Model file for the job. Use its own axes, mm. A direction names the side the tool comes from. Give positions to 0.01 mm unless a question says otherwise; leave off trailing zeros. Write each loop counter-clockwise with the first axis right and the second up, starting at its lowest first coordinate (ties: lowest second). Pieces come first, ordered by that corner, then holes.
```python
from build123d import *

# Parameters (mm, degrees)
SKETCH1_R             = 10.5
SKETCH1_R_2           = 3
EXTRUDE1_DEPTH        = 46.5
SKETCH1_3_R           = 3
CUT_EXTRUDE1_DEPTH    = 49.813420286
CUT_EXTRUDE4_DEPTH    = 8.5
CUT_EXTRUDE6_START    = -37
SKETCH6_R             = 10.5
SKETCH6_R_2           = 6
CUT_EXTRUDE6_DEPTH    = 37
CUT_EXTRUDE7_START    = -1
SKETCH7_R             = 10.5
SKETCH7_R_2           = 7.5
CUT_EXTRUDE7_DEPTH    = 1
M4X0_7_TAPPED_HOLE1_D = 3
SKETCH8_OUTSIDE_W     = 33.82
SKETCH8_OUTSIDE_H     = 30.82
CUT_EXTRUDE8_DEPTH    = 30
FILLET1_R             = 0.5
CHAMFER1_SIZE         = 0.5
FILLET2_R             = 0.3
CHAMFER2_SIZE         = 1


with BuildPart() as part:
    # Sketch1 → Extrude1 (new body)
    # profile 1 of 2: a face of its own
    with BuildSketch(Plane.XY):
        Circle(SKETCH1_R)
        Circle(SKETCH1_R_2, mode=Mode.SUBTRACT)
    # profile 2 of 2: a face of its own
    with BuildSketch(Plane.XY):
        Circle(SKETCH1_R_2)
    extrude(amount=-EXTRUDE1_DEPTH)

    # Sketch1<3> → Cut-Extrude1 (cut, through all)
    with BuildSketch(Plane.XY):
        Circle(SKETCH1_3_R)
    extrude(amount=-CUT_EXTRUDE1_DEPTH, mode=Mode.SUBTRACT)

    # Sketch4 → Cut-Extrude4 (cut)
    with BuildSketch(Plane.XY):
        with BuildLine():
            Line((-10.24499878, 2.3), (10.24499878, 2.3))
            ThreePointArc((10.24499878, 2.3), (0, 10.5), (-10.24499878, 2.3))
        make_face()
    extrude(amount=-CUT_EXTRUDE4_DEPTH, mode=Mode.SUBTRACT)

    # Sketch6 → Cut-Extrude6 (cut)
    with BuildSketch(Plane(origin=(0, 0, -46.5), x_dir=(1, 0, 0), z_dir=(0, 0, -1)).offset(CUT_EXTRUDE6_START)):
        Circle(SKETCH6_R)
        with Locations(Location((0, 0, 0), (0, 0, 270))):
            Circle(SKETCH6_R_2, mode=Mode.SUBTRACT)
    extrude(amount=CUT_EXTRUDE6_DEPTH, mode=Mode.SUBTRACT)

    # Sketch7 → Cut-Extrude7 (cut)
    with BuildSketch(Plane(origin=(0, 0, -9.5), x_dir=(1, 0, 0), z_dir=(0, 0, -1)).offset(CUT_EXTRUDE7_START)):
        Circle(SKETCH7_R)
        with Locations(Location((0, 0, 0), (0, 0, 270))):
            Circle(SKETCH7_R_2, mode=Mode.SUBTRACT)
    extrude(amount=CUT_EXTRUDE7_DEPTH, mode=Mode.SUBTRACT)

    # M4x0.7 Tapped Hole1 (through all)
    with Locations(Plane(origin=(6.25, 2.3, -4.25), x_dir=(0, 0, 1), z_dir=(0, 1, 0))):
        with Locations((0, 0), (0, -12.5)):
            Hole(M4X0_7_TAPPED_HOLE1_D / 2)

    # Sketch8 outside → Cut-Extrude8 (cut)
    with BuildSketch(Plane(origin=(0, 0, -46.5), x_dir=(1, 0, 0), z_dir=(0, 0, -1))):
        with Locations((0, 1.5)):
            Rectangle(SKETCH8_OUTSIDE_W, SKETCH8_OUTSIDE_H)
        Polygon((0, 5.773502692), (-5, 2.886751346), (-5, -2.886751346), (0, -5.773502692), (5, -2.886751346), (5, 2.886751346), align=None, mode=Mode.SUBTRACT)
    extrude(amount=-CUT_EXTRUDE8_DEPTH, mode=Mode.SUBTRACT)

    # Fillet1
    fillet1_edges = [part.edges().sort_by_distance(p)[0] for p in [
        (5, -2.886751346, -31.5),
        (5, 2.886751346, -31.5),
        (0, 5.773502692, -31.5),
        (-5, 2.886751346, -31.5),
        (-5, -2.886751346, -31.5),
        (0, -5.773502692, -31.5),
    ]]
    fillet(fillet1_edges, radius=FILLET1_R)

    # Chamfer1
    chamfer1_edges = [part.edges().sort_by_distance(p)[0] for p in [
        (-2.5, -4.330127019, -46.5),
        (2.5, -4.330127019, -46.5),
        (-5, 0, -46.5),
        (-2.5, 4.330127019, -46.5),
        (2.5, 4.330127019, -46.5),
        (5, 0, -46.5),
        (0, -5.696152423, -46.5),
        (4.933012702, -2.848076211, -46.5),
        (4.933012702, 2.848076211, -46.5),
        (0, 5.696152423, -46.5),
        (-4.933012702, 2.848076211, -46.5),
        (-4.933012702, -2.848076211, -46.5),
    ]]
    chamfer(chamfer1_edges, length=CHAMFER1_SIZE - 0.0001)  # a hair under: the kernel refuses the full size

    # Sketch12 → Groove for ANSI B27.7 - 3AM1-12, Basic External Retaining Ring1 (revolve, cut)
    with BuildSketch(Plane(origin=(0, 0, 19.370057685), x_dir=(0, 1, 0), z_dir=(-1, 0, 0))):
        with BuildLine():
            Line((5.775, 33.970057685), (7.275, 33.970057685))
            Line((7.275, 33.970057685), (7.275, 35.070057685))
            Line((7.275, 35.070057685), (5.775, 35.070057685))
            ThreePointArc((5.775, 35.070057685), (5.704289322, 35.040768363), (5.675, 34.970057685))
            Line((5.675, 34.970057685), (5.675, 34.070057685))
            ThreePointArc((5.675, 34.070057685), (5.704289322, 33.999347007), (5.775, 33.970057685))
        make_face()
    revolve(axis=Axis((0, 0, 69.359173663), (0, 0, -1)), mode=Mode.SUBTRACT)

    # Fillet2
    fillet2_edges = [part.edges().sort_by_distance(p)[0] for p in [
        (0, -6, -9.5),
        (0, -7.5, -8.5),
    ]]
    fillet(fillet2_edges, radius=FILLET2_R)

    # Chamfer2
    chamfer2_edges = [part.edges().sort_by_distance(p)[0] for p in [
        (0, -10.5, 0),
        (0, -10.5, -8.5),
    ]]
    chamfer(chamfer2_edges, length=CHAMFER2_SIZE)


solid = part.part
```
1. Slice it at A-A, the plane z = -20.5. Write the cut outline in (x, y), and give its area (3 significant figures).
Calculated:
outline: (-5, -2.6) arc R0.5 ccw to (-4.75, -3.03) - (-0.25, -5.63) arc R0.5 ccw to (0.25, -5.63) - (4.75, -3.03) arc R0.5 ccw to (5, -2.6) - (5, 2.6) arc R0.5 ccw to (4.75, 3.03) - (0.25, 5.63) arc R0.5 ccw to (-0.25, 5.63) - (-4.75, 3.03) arc R0.5 ccw to (-5, 2.6) - close; hole circle Ø6 at (0, 0)
area: 58.2 mm2
2. Pin check, flat tips, straight feed: P1, Ø6, axis at y = 0.5, z = -24.5, coming from the +X side; P2, Ø1.6, axis at x = 0.5, y = 4.5, coming from the +Z side; P3, Ø10, axis at x = 5, z = -32.5, coming from the +Y side. Stop position of each tip, or through.
Calculated:
P1: stops at x = 5
P2: stops at z = -8.5
P3: stops at y = 5.7
3. Which spindle directions (+Z, -Z, +X, -X, +Y, -Y) get a long thin tool onto all of the face, cutting with end or side? Do faces 1 (the cylindrical face through (-2.174, 5.242, -15.144)), 2 (the cylindrical face through (1.802, 5.723, -16.094)), 3 (the flat face through (-5, 0, -31)), 4 (the flat face through (0, 4, -8.5)), 5 (the flat face through (-2.469, -4.348, -31.457)). Say none if no direction does.
Calculated:
face 1: none
face 2: -Z
face 3: -Z, -X, +Y, -Y
face 4: +Z, +X, -X, +Y
face 5: -Z, -X, -Y
4. Slice it at B-B, the plane y = 0. State how many separate pieces and enclosed holes the cut face has, and give its area (3 significant figures).
Calculated:
separate pieces: 2
enclosed holes: 2
area: 281 mm2
5. Probe probe 1 along X at (y, z) = (0, -10.5); probe 2 along Z at (x, y) = (6.25, -2.5); probe 3 along X at (y, z) = (-3.5, -4.25). List the from-to ranges inside material, lowest first.
Calculated:
probe 1: x = -6 to -3, 3 to 6
probe 2: z = -9.5 to -5.75, -2.75 to 0
probe 3: x = -9.9 to -7.75, -4.75 to 4.75, 7.75 to 9.9
6. Pull direction X, two halves, no side cores. Call faces 6 (the cylindrical face through (-0.65, -2.93, -22.92)), 7 (the flat face through (-2, -8, -8.5)), 8 (the cylindrical face through (-2.87, 6.93, -9.1)), 9 (the flat face through (-2.408, 4.099, -46.247)): +X half, -X half, draft (parallel to the pull), parting line (faces both ways), or undercut.
Calculated:
face 6: undercut
face 7: draft
face 8: parting line
face 9: -X half
7. Slice it at C-C, the plane z = -4.25. Write the cut outline in (x, y) (3 decimals).
Calculated:
outline: (-10.245, 2.3) arc R10.5 ccw to (-7.75, -7.084) - (-7.75, 2.3) - close; (-4.75, -9.364) arc R10.5 ccw to (4.75, -9.364) - (4.75, 2.3) - (1.926, 2.3) arc R3 cw (long way) to (-1.926, 2.3) - (-4.75, 2.3) - close; (7.75, -7.084) arc R10.5 ccw to (10.245, 2.3) - (7.75, 2.3) - close
8. Slice it at D-D, the plane z = -10.5. Write the cut outline in (x, y), and give its area (3 significant figures).
Calculated:
outline: circle Ø12 at (0, 0); hole circle Ø6 at (0, 0)
area: 84.8 mm2
